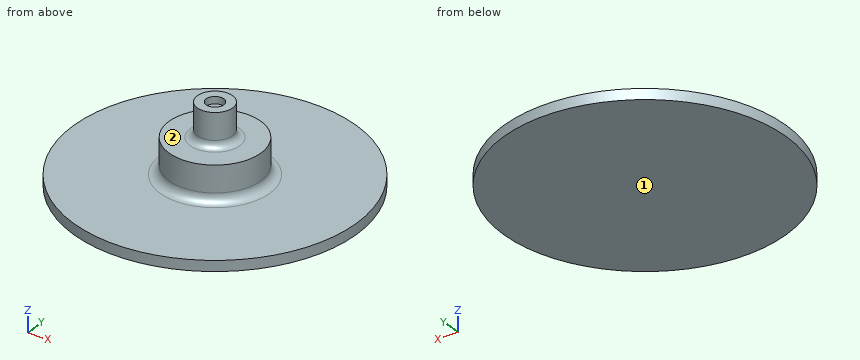
Autodesk Fusion 360 part; units mm, degrees
sketch "Sketch1" plane through (0, 0, 0) normal (0, 0, 1) x (1, 0, 0)
  circle A0 centre (0, 0) radius 2.5
  circle A1 centre (0, 0) radius 5
  dimension "d1" = 5
  dimension "d2" = 10
extrude "Extrude1" add sketch "Sketch1" along normal blind 2
extrude "Extrude2" add sketch "Sketch1" against normal blind 5.5 contours A0 | A1
sketch "Sketch2" plane through (0, 0, -5.5) normal (0, 0, -1) x (1, 0, 0)
  circle A0 centre (0, 0) radius 5
  circle A1 centre (0, 0) radius 13
  dimension "d7" = 26
extrude "Extrude3" add sketch "Sketch2" along normal blind 5 contours A0 | A1
extrude "Extrude4" cut 1 faces at (10.2663, 0.8943, -5.5) along direction (0, 0, -1) blind 2
fillet "Fillet1" radius 2 1 edges at (-4.6616, -1.8081, -7.5)
extrude "Extrude5" add 1 faces at (2.1667, -3.7528, -10.5) along direction (0, 0, -1) blind 5.5
extrude "Extrude6" add 1 faces at (2.1667, -3.7528, -16) along direction (0, 0, -1) blind 1.5
sketch "Sketch3" plane through (0, 0, -17.5) normal (0, 0, -1) x (1, 0, 0)
  circle A0 centre (0, 0) radius 13
  circle A1 centre (0, 0) radius 40
  dimension "d18" = 80
extrude "Extrude7" add sketch "Sketch3" along normal blind 3 contours A0 | A1
fillet "Fillet2" radius 2.5 1 edges at (-12.1203, 4.701, -17.5)
Read the model definition and answer for the solid it produces. Units are mm, in the model's axes. Face numbers are marked on the shaded views. A direction names the side the tool comes from. Coordinates: 2 decimals unless noted, no trailing zeros. Write each loop counter-clockwise with the first axis right and the second up, starting at its lowest first coordinate (ties: lowest second). Pieces come first, ordered by that corner, then holes. Notation, with made-up numbers: (53, -8) -> (107, -8) arc R15 cw to (107, 12) -> close; hole circle Ø6 at (-7, 9.25). An arc over 180 degrees is marked (long way). Answer as a JSON object with one key per item and string values.
Q1. The part is cut by section D-D on y = -22. Give the vertices of the cut face in (x, z).
The answers:
{"outline": "(-33.41, -20.5) -> (33.41, -20.5) -> (33.41, -17.5) -> (-33.41, -17.5) -> close"}
Q2. Consider line 1 (Y direction, x = 0, z = 1.5); line 2 (Z direction, x = 18.5, y = -31.5); line 3 (Y direction, x = 0, z = -3.75). Determine where each line is inside the solid, lowest interval first. Write a range as [from, to].
The answers:
{"line 1": "y = [-5, -2.5], [2.5, 5]", "line 2": "z = [-20.5, -17.5]", "line 3": "y = [-5, 5]"}
Q3. Flat-ended cylindrical pins translate along their axes: pin 1 Ø8 at (x, z) = (-0.5, -8.5) entering from -Y; pin 2 Ø3 at (y, z) = (4.5, -7) entering from -X; pin 3 Ø1.5 at (x, y) = (10.5, -11.5) entering from +Z; pin 4 Ø5.5 at (x, y) = (0, -1) entering from +Z. Find the tip coordinate at first contact, or state that the pin passes through.
The answers:
{"pin 1": "stops at y = -13", "pin 2": "stops at x = -12.63", "pin 3": "stops at z = -17.41", "pin 4": "stops at z = 2"}
Q4. A tool of negligible diameter and unlimited length cuts with its end or side. For the marked faces 1 and 2, from which of +Z, -Z, +X, -X, +Y, -Y can it reach the whole face along a straight path? Write none if from no direction.
The answers:
{"face 1": "-Z, +X, -X, +Y, -Y", "face 2": "+Z"}
Q5. The part is cut by section A-A on y = 0. Give the vertices of the cut face in (x, z), then the cut area to 3 significant figures.
The answers:
{"outline": "(-40, -20.5) -> (40, -20.5) -> (40, -17.5) -> (15.5, -17.5) arc R2.5 cw to (13, -15) -> (13, -7.5) -> (7, -7.5) arc R2 cw to (5, -5.5) -> (5, 2) -> (2.5, 2) -> (2.5, 0) -> (-2.5, 0) -> (-2.5, 2) -> (-5, 2) -> (-5, -5.5) arc R2 cw to (-7, -7.5) -> (-13, -7.5) -> (-13, -15) arc R2.5 cw to (-15.5, -17.5) -> (-40, -17.5) -> close", "area": "589 mm2"}
Q6. The part is cut by section C-C on z = -12.75. Give the vertices of the cut face in (x, y).
The answers:
{"outline": "circle Ø26 at (0, 0)"}
